Here's the drawing with two shaded views (mm, measured from the low corner). I have some questions. A direction names the side the tool comes from. Give positions to 0.01 mm unless a question says otherwise; leave off trailing zeros. Write each loop counter-clockwise with the first axis right and the second up, starting at its lowest first coordinate (ties: lowest second). Pieces come first, ordered by that corner, then holes.
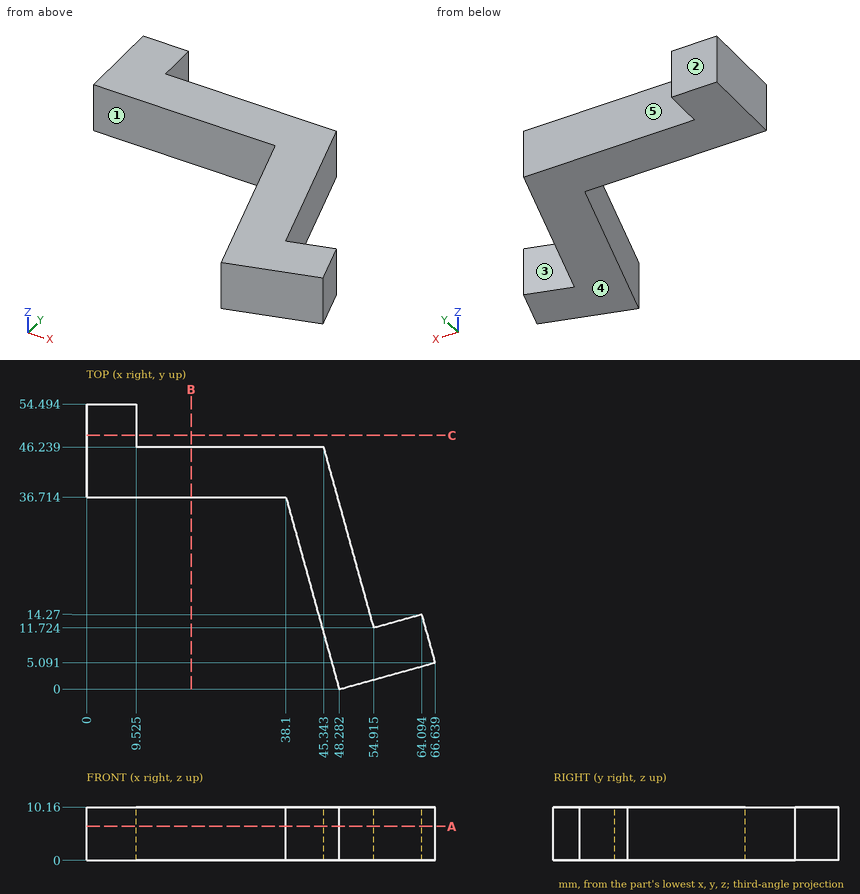
(1) For the marked faces 1, 2, 3, 4 and 5, which set-ups out of +Z, -Z, +X, -X, +Y, -Y let a thin tool reach every point of the face, with its end or its side?
Returned:
face 1: +Z, -Z, -X, -Y
face 2: +Z, -Z, +X, -X, +Y
face 3: +Z, -Z, +Y
face 4: -Z, +X, -X, +Y, -Y
face 5: +Z, -Z, +X, +Y
(2) Will these pins go through, and if not, where does the flat tip stop? P1, Ø2, axis at x = 43, z = 6.5, coming from the +Y side; P2, Ø5, axis at x = 9.5, z = 4.5, coming from the -Y side; P3, Ø1, axis at y = 11.5, z = 6.5, coming from the -X side.
Returned:
P1: stops at y = 46.24
P2: stops at y = 36.71
P3: stops at x = 44.95
(3) If I drill on L1, parallel to Y at x = 38, z = 8 (1 decimal); L2, parallel to X at y = 49.5, z = 2.5 (1 decimal); L3, parallel to Y at x = 3.5, z = 3.5 (1 decimal), over which ranges is the centre line in solid material (lowest first)?
Returned:
L1: y = 36.7 to 46.2
L2: x = 0 to 9.5
L3: y = 36.7 to 54.5
(4) Imagine slicing it at C-C, the plane y = 48.5. Write out the boundary of the cut face in (x, z) (1 decimal).
Returned:
outline: (0, 0) - (9.5, 0) - (9.5, 10.2) - (0, 10.2) - close
(5) Imagine slicing it at B-B, the plane x = 20. Write out the boundary of the cut face in (y, z) (1 decimal).
Returned:
outline: (36.7, 0) - (46.2, 0) - (46.2, 10.2) - (36.7, 10.2) - close
(6) Imagine slicing it at A-A, the plane z = 6.5. Write out the boundary of the cut face in (x, y) (1 decimal), plus the area to 3 significant figures.
Returned:
outline: (0, 36.7) - (38.1, 36.7) - (48.3, 0) - (66.6, 5.1) - (64.1, 14.3) - (54.9, 11.7) - (45.3, 46.2) - (9.5, 46.2) - (9.5, 54.5) - (0, 54.5) - close
area: 964 mm2
